The listing builds one solid part. Answer for the finished solid, in the listing's coordinates (mm). Give positions to 0.01 mm unless a question says otherwise; leave off trailing zeros. Order: outer loops, then holes, each group sorted by start corner. A loop starts at its lowest first (then second) coordinate and runs counter-clockwise, first axis right, second up. Notation, with made-up numbers: (57, 54.5) - (105, 54.5) arc R33 ccw to (105, 87.5) - close; hole circle Ø3 at (29, 29.5). An arc over 180 degrees is marked (long way). Answer in a Markdown table with one row per item.
Autodesk Inventor part; units mm, degrees
ref_plane "YZ Plane" through (0, 0, 0) normal (1, 0, 0) x (0, 1, 0)
ref_plane "XZ Plane" through (0, 0, 0) normal (0, 1, 0) x (-1, 0, 0)
ref_plane "XY Plane" through (0, 0, 0) normal (0, 0, 1) x (1, 0, 0)
sketch "Sketch1" plane through (0, 0, 0) normal (0, 0, 1) x (1, 0, 0)
  line L0 (-285, 285) -> (285, 285)
  line L1 (285, 285) -> (285, -285)
  line L2 (285, -285) -> (-285, -285)
  line L3 (-285, -285) -> (-285, 285)
  line L4 (-285, 285) -> (285, -285) construction
  line L5 (285, 285) -> (-285, -285) construction
  line L6 (-246.5, -246.5) -> (246.5, -246.5)
  line L7 (246.5, -246.5) -> (246.5, 246.5)
  line L8 (246.5, 246.5) -> (-246.5, 246.5)
  line L9 (-246.5, 246.5) -> (-246.5, -246.5)
  line L10 (-246.5, -246.5) -> (246.5, 246.5) construction
  line L11 (246.5, -246.5) -> (-246.5, 246.5) construction
  line L12 (-246.5, 246.5) -> (-285, 285)
  line L13 (246.5, -246.5) -> (285, -285)
  point P0 (0, 0)
  dimension "d1" = 570
  dimension "d2" = 493
extrude "Plate1" add sketch "Sketch1" along normal blind 2 contours L0 L1 L13 L7 L8 L12
chamfer "Corner Chamfer1" distance 1 angle 45 2 edges at (-285, 285, 1) (285, -285, 1)
sketch "Sketch2" plane through (0, 0, 0) normal (0, 0, -1) x (-1, 0, 0)
  line L0 (-284.2929, -284.2929) -> (-285, -284)
  line L1 (-246.5, -246.5) -> (-284.2929, -284.2929)
  line L2 (-246.5, 246.5) -> (-246.5, -246.5) construction
  line L3 (246.5, 246.5) -> (-246.5, 246.5) construction
  line L4 (284.2929, 284.2929) -> (246.5, 246.5)
  line L5 (284, 285) -> (284.2929, 284.2929)
  line L6 (-285, 285) -> (284, 285) construction
  line L7 (-285, -284) -> (-285, 285) construction
  circle A0 centre (-275, 240.5) radius 2.75
  circle A1 centre (-275, 80.5) radius 2.75
  circle A2 centre (-275, -79.5) radius 2.75
  circle A3 centre (-275, -239.5) radius 2.75
  line L8 (-275, 285) -> (-275, -275) construction
  line L9 (-285, 275) -> (275, 275) construction
  line L10 (-285, -284) -> (-285, 285) construction
  circle A4 centre (-205, 275) radius 2.75
  circle A5 centre (-5, 275) radius 2.75
  circle A6 centre (195, 275) radius 2.75
  point P0 (0, 0)
  point P1 (-285, 0.5)
  point P2 (-285, 0.5)
  point P3 (-285, 0.5)
  point P4 (-285, 0.5)
  dimension "d7" = 5.5
  dimension "d8" = 10
  dimension "d9" = 10
  dimension "d10" = 80
  dimension "d11" = 80
  dimension "d12" = 240
  dimension "d13" = 240
  dimension "d14" = 200
  dimension "d15" = 200
extrude "Cut1" cut sketch "Sketch2" against normal blind 2
equation "\"d9\" = d8"
equation "\"d15\" = d14"
equation "\"d16\" = Thickness"
equation "\"d3\" = Thickness"
equation "\"BendRadius\" = Thickness"
equation "\"BendReliefWidth\" = Thickness"
equation "\"BendReliefDepth\" = 0.5 * Thickness"
equation "\"CornerReliefSize\" = 4 * Thickness"
equation "\"MinimumRemnant\" = 2 * Thickness"
equation "\"TransitionRadius\" = BendRadius"
equation "\"JacobiRadiusSize\" = BendRadius"
equation "\"GapSize\" = Thickness"
properties part number "PNS waste water bin 01"
Item 1: This flat-tipped pin is pushed along its axis until it touches: P1, Ø3.5, axis at x = 275, y = -239.5, coming from the +Z side. Where does it stop, or does it pass through?
Answer block:
| item | result |
|---|---|
| P1 | through |
Item 2: Find section B-B on y = -130. Write down the section's boundary in (x, z), then the cut area to 3 significant figures.
Answer block:
| item | result |
|---|---|
| outline | (246.5, 0) - (285, 0) - (285, 2) - (246.5, 2) - close |
| area | 77.0 mm² |
Item 3: Consider line 1 (Y direction, x = -195, z = 1.1); line 2 (X direction, y = 275, z = 0.85); line 3 (Y direction, x = 275, z = 1.05). Determine where each line is inside the solid, lowest interval first.
Answer block:
| item | result |
|---|---|
| line 1 | 246.5 to 272.25, 277.75 to 285 |
| line 2 | -275 to -197.75, -192.25 to 2.25, 7.75 to 202.25, 207.75 to 285 |
| line 3 | -275 to -242.25, -236.75 to -82.25, -76.75 to 77.75, 83.25 to 237.75, 243.25 to 285 |
Item 4: Find section A-A on z = 1.2. Write down the section's boundary in (x, y).
Answer block:
| item | result |
|---|---|
| outline | (-284.29, 284.29) - (-246.5, 246.5) - (246.5, 246.5) - (246.5, -246.5) - (284.29, -284.29) - (285, -284) - (285, 285) - (-284, 285) - close; hole circle Ø5.5 at (-195, 275); hole circle Ø5.5 at (5, 275); hole circle Ø5.5 at (205, 275); hole circle Ø5.5 at (275, -239.5); hole circle Ø5.5 at (275, -79.5); hole circle Ø5.5 at (275, 80.5); hole circle Ø5.5 at (275, 240.5) |
